Part model, mm, in its own coordinate system. A direction names the side the tool comes from. Coordinates: 2 decimals unless noted, no trailing zeros. Order: outer loops, then holes, each group sorted by start corner. A loop starts at its lowest first (then second) coordinate and runs counter-clockwise, first axis right, second up.
```python
from build123d import *

# Parameters (mm, degrees)
SKETCH1_W                 = 95.25
SKETCH1_H                 = 76.2
BOSS_EXTRUDE1_DEPTH       = 4.7625
F_8_CLEARANCE_HOLE1_D     = 4.9149
FILLET1_R                 = 2.54
F_8_CLEARANCE_SLOT1_DEPTH = 4.7625
SKETCH6_R                 = 4.064
CUT_EXTRUDE1_DEPTH        = 62.175420156


# Read off the part's stored shape, not the designer's step: #8 Clearance Slot1
with BuildPart() as part:
    # Sketch1 → Boss-Extrude1 (new body)
    with BuildSketch(Plane.XY):
        Rectangle(SKETCH1_W, SKETCH1_H)
    extrude(amount=BOSS_EXTRUDE1_DEPTH)

    # #8 Clearance Hole1 (through all)
    with Locations(Plane.XY.offset(4.7625)):
        with Locations((23.57, 23.57), (-23.57, 23.57), (-23.57, -23.57), (23.57, -23.57)):
            Hole(F_8_CLEARANCE_HOLE1_D / 2)

    # Fillet1
    fillet1_edges = [part.edges().sort_by_distance(p)[0] for p in [
        (-47.625, 38.1, 2.38125),
        (47.625, 38.1, 2.38125),
        (47.625, -38.1, 2.38125),
        (-47.625, -38.1, 2.38125),
    ]]
    fillet(fillet1_edges, radius=FILLET1_R)

    # #8 Clearance Slot1 outline → #8 Clearance Slot1 (cut)
    with BuildSketch(Plane.XY):
        with BuildLine():
            ThreePointArc((-40.1604, 21.2979), (-37.9125, 19.05), (-35.6646, 21.2979))
            Line((-35.6646, 21.2979), (-35.6646, 29.5021))
            ThreePointArc((-35.6646, 29.5021), (-37.9125, 31.75), (-40.1604, 29.5021))
            Line((-40.1604, 29.5021), (-40.1604, 21.2979))
        make_face()
        with BuildLine():
            ThreePointArc((-35.6646, -21.2979), (-37.9125, -19.05), (-40.1604, -21.2979))
            Line((-40.1604, -21.2979), (-40.1604, -29.5021))
            ThreePointArc((-40.1604, -29.5021), (-37.9125, -31.75), (-35.6646, -29.5021))
            Line((-35.6646, -29.5021), (-35.6646, -21.2979))
        make_face()
        with BuildLine():
            ThreePointArc((35.6646, -29.5021), (37.9125, -31.75), (40.1604, -29.5021))
            Line((40.1604, -29.5021), (40.1604, -21.2979))
            ThreePointArc((40.1604, -21.2979), (37.9125, -19.05), (35.6646, -21.2979))
            Line((35.6646, -21.2979), (35.6646, -29.5021))
        make_face()
        with BuildLine():
            ThreePointArc((40.1604, 29.5021), (37.9125, 31.75), (35.6646, 29.5021))
            Line((35.6646, 29.5021), (35.6646, 21.2979))
            ThreePointArc((35.6646, 21.2979), (37.9125, 19.05), (40.1604, 21.2979))
            Line((40.1604, 21.2979), (40.1604, 29.5021))
        make_face()
    extrude(amount=F_8_CLEARANCE_SLOT1_DEPTH, mode=Mode.SUBTRACT)

    # Sketch6 → Cut-Extrude1 (cut, through all)
    with BuildSketch(Plane(origin=(0, 0, 0), x_dir=(-1, 0, 0), z_dir=(0, 0, -1))):
        with Locations((-37.9125, 21.2979)):
            Circle(SKETCH6_R)
        with Locations((-37.9125, -29.5021)):
            Circle(SKETCH6_R)
        with Locations((37.9125, -29.5021)):
            Circle(SKETCH6_R)
        with Locations((37.9125, 21.2979)):
            Circle(SKETCH6_R)
    extrude(amount=-CUT_EXTRUDE1_DEPTH, mode=Mode.SUBTRACT)


solid = part.part
```
(1) Slice it at D-D, the plane y = 23.57. Give the cut face in (x, z) (1 decimal).
(2) Tool access for faces 5 (the face through (37.96, -19.05, 2.35)), 6 (the face through (-46.901, -37.336, 2.415)): list every direction of +Z, -Z, +X, -X, +Y, -Y with a clear straight run to the whole face (end or side of a thin tool).
(3) Slice it at A-A, the plane x = 23.57. Give the cut face in (y, z), then the cut area to 3 significant figures.
(4) Drop a flat-ended pin along its axis: pin 1 (5 mm diameter, centred on x = -37.91, y = -29.5, fed in from +Z). Give the stop position or say it passes through.
(5) Pull direction X, two halves, no side cores. Call faces 1 (the face through (46.861, -37.376, 2.415)), 2 (the face through (-46.901, 37.336, 2.415)), 3 (the face through (-35.665, -24, 2)), 4 (the face through (35.665, 27, 2)): +X half, -X half, draft (parallel to the pull), parting line (faces both ways), or undercut.
(6) Slice it at C-C, the plane y = -23.57. Give the cut face in (x, z) (1 decimal), then the cut area to 3 significant figures.
(7) Probe line 1 (Y direction, x = -23.57, z = 1.6); line 2 (X direction, y = 29.5, z = 2.6) (3 decimals); line 3 (X direction, y = -23.5, z = 3.8) (3 decimals). List the from-to ranges inside material, lowest first.
(8) Slice it at B-B, the plane z = 3.45. State how many separate pieces and enclosed holes the cut face has, then the cut area to 3 significant figures.
Here are the results:
1. outline: (-47.6, 0) - (-41.3, 0) - (-41.3, 4.8) - (-47.6, 4.8) - close; (-34.5, 0) - (-26, 0) - (-26, 4.8) - (-34.5, 4.8) - close; (-21.1, 0) - (21.1, 0) - (21.1, 4.8) - (-21.1, 4.8) - close; (26, 0) - (34.5, 0) - (34.5, 4.8) - (26, 4.8) - close; (41.3, 0) - (47.6, 0) - (47.6, 4.8) - (41.3, 4.8) - close
2. face 5: +Z, -Z
2. face 6: +Z, -Z, -X, -Y
3. outline: (-38.1, 0) - (-26.03, 0) - (-26.03, 4.76) - (-38.1, 4.76) - close; (-21.11, 0) - (21.11, 0) - (21.11, 4.76) - (-21.11, 4.76) - close; (26.03, 0) - (38.1, 0) - (38.1, 4.76) - (26.03, 4.76) - close
3. area: 316 mm2
4. pin 1: passes through
5. face 1: +X half
5. face 2: -X half
5. face 3: undercut
5. face 4: undercut
6. outline: (-47.6, 0) - (-40.2, 0) - (-40.2, 4.8) - (-47.6, 4.8) - close; (-35.7, 0) - (-26, 0) - (-26, 4.8) - (-35.7, 4.8) - close; (-21.1, 0) - (21.1, 0) - (21.1, 4.8) - (-21.1, 4.8) - close; (26, 0) - (35.7, 0) - (35.7, 4.8) - (26, 4.8) - close; (40.2, 0) - (47.6, 0) - (47.6, 4.8) - (40.2, 4.8) - close
6. area: 364 mm2
7. line 1: y = -38.1 to -26.03, -21.11 to 21.11, 26.03 to 38.1
7. line 2: x = -47.625 to -40.16, -35.665 to 35.665, 40.16 to 47.625
7. line 3: x = -47.625 to -40.16, -35.665 to -26.026, -21.114 to 21.114, 26.026 to 35.665, 40.16 to 47.625
8. separate pieces: 1
8. enclosed holes: 8
8. area: 6,860 mm2
